```python
from build123d import *

# Parameters (mm, degrees)
SKETCH2_W           = 38.1
SKETCH2_H           = 25.4
BOSS_EXTRUDE1_DEPTH = 76.2
SKETCH3_W           = 19.05
SKETCH3_H           = 25.4
REVOLVE1_ANGLE      = 180
SKETCH4_R           = 4.7625
CUT_EXTRUDE1_DEPTH  = 101.40231571


with BuildPart() as part:
    # Sketch2 → Boss-Extrude1 (new body)
    with BuildSketch(Plane(origin=(0, 0, 0), x_dir=(1, 0, 0), z_dir=(0, 1, 0))):
        Rectangle(SKETCH2_W, SKETCH2_H)
    extrude(amount=BOSS_EXTRUDE1_DEPTH)

    # Sketch3 → Revolve1 (revolve)
    with BuildSketch(Plane(origin=(0, 76.2, 0), x_dir=(1, 0, 0), z_dir=(0, 1, 0))):
        with Locations((9.525, 0)):
            Rectangle(SKETCH3_W, SKETCH3_H)
    revolve(axis=Axis((0, 76.2, -12.7), (0, 0, 1)), revolution_arc=REVOLVE1_ANGLE)

    # Sketch4 → Cut-Extrude1 (cut, through all)
    with BuildSketch(Plane.XY.offset(12.7)):
        with Locations((0, 76.2)):
            Circle(SKETCH4_R)
    extrude(amount=-CUT_EXTRUDE1_DEPTH, mode=Mode.SUBTRACT)


solid = part.part
```
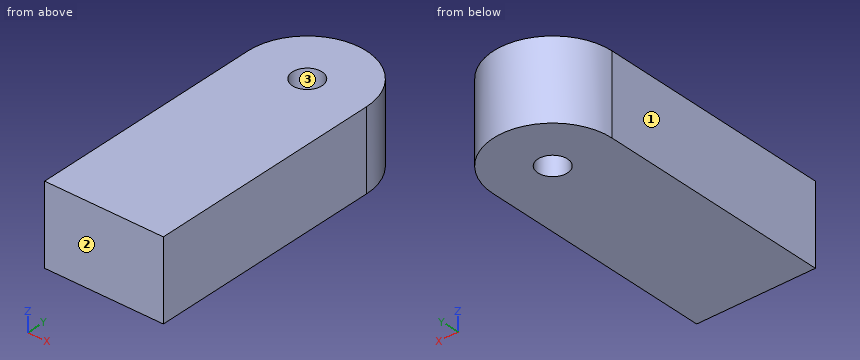
For this review, take the finished solid that the model builds, in its own axes (mm). Face numbers are marked on the shaded views. Round coordinates to 2 decimals unless told otherwise and drop trailing zeros. Loops run counter-clockwise (first coordinate to the right, second up) from the corner with the lowest first, then second, coordinate; pieces in that order, holes last.
Q1. Add section D-D on x = 14.5. Write out the cut boundary in (y, z).
Result sheet:
outline: (0, -12.7) - (88.56, -12.7) - (88.56, 12.7) - (0, 12.7) - close
Q2. To check wall thickness, follow line 1 along X through (y, z) = (76, 9.75); line 2 along Y through (x, z) = (0, -7.5); line 3 along X through (y, z) = (74, 2.25). State the ranges of each line that lie inside material, in increasing order.
Result sheet:
line 1: x = -19.05 to -4.76, 4.76 to 19.05
line 2: y = 0 to 71.44, 80.96 to 95.25
line 3: x = -19.05 to -4.22, 4.22 to 19.05
Q3. Add section A-A on x = 0. Write out the cut boundary in (y, z), plus the area to 3 significant figures.
Result sheet:
outline: (0, -12.7) - (71.44, -12.7) - (71.44, 12.7) - (0, 12.7) - close; (80.96, -12.7) - (95.25, -12.7) - (95.25, 12.7) - (80.96, 12.7) - close
area: 2,180 mm2
Q4. Add section C-C on x = -16. Write out the cut boundary in (y, z).
Result sheet:
outline: (0, -12.7) - (86.54, -12.7) - (86.54, 12.7) - (0, 12.7) - close
Q5. Mouldability with a two-part tool opening along X and no side actions: class the marked faces 1, 2 and 3 as +X half, -X half, draft (parallel to the pull), parting line (faces both ways), or undercut.
Result sheet:
face 1: -X half
face 2: draft
face 3: undercut
Q6. Insertion check: pin 1 Ø1 at (x, z) = (4.5, 3.5) entering from +Y; pin 2 Ø5.5 at (x, y) = (0, 76.2) entering from +Z. Each pin has a flat end and moves straight along its axis. Give the tip position at first contact, or say it passes through.
Result sheet:
pin 1: stops at y = 94.83
pin 2: passes through
